Check sheet for the modelled part. Datum: model origin and axes. Units: mm. A direction names the side the tool comes from. Give positions to 0.01 mm unless a question says otherwise; leave off trailing zeros. Loops run counter-clockwise (first coordinate to the right, second up) from the corner with the lowest first, then second, coordinate; pieces in that order, holes last. Notation, with made-up numbers: (-8.75, 66) - (15.25, 66) arc R26 cw to (15.25, 101) - close; hole circle Ø1 at (27.25, 85.5). An arc over 180 degrees is marked (long way). Answer in a Markdown table with one row per item. Add a question column.
(1) Thickness scan on L1, parallel to Y at x = 0, z = -2.25; L2, parallel to Y at x = 0, z = 3.8; L3, parallel to Z at x = -14.75, y = 0. Record the ranges inside material, lowest first.
(2) Sectioned sample at C-C on z = 0.5. Enter the section's corners in (x, y), then the cut area to 3 significant figures.
(3) Set-up check for faces 1 (the face through (-2.39, -10.36, -4.93)), 2 (the face through (0.37, 7.34, 2.46)): record each of +Z, -Z, +X, -X, +Y, -Y from which the full face is reachable in a straight line by a thin tool's end or side.
(4) Go/stop test with flat-tipped pins: P1, Ø6, axis at x = -6, z = -4.5, coming from the -Y side; P2, Ø0.7, axis at x = -6, y = 1, coming from the -Z side; P3, Ø0.7, axis at x = -7, z = -5, coming from the -Y side. Record where each tip stops, or that it passes through.
(5) Draft check along Y on faces 3 (the face through (4, 0, -10)), 4 (the face through (2.39, 10.36, -4.93)). Enter one of: released by +Y, released by -Y, zero draft, split by the parting line, or undercut.
(6) Sectioned sample at A-A on y = 0. State how many separate pieces and enclosed holes the cut face has, then the cut area to 3 significant figures.
(7) Sectioned sample at B-B on x = 0. Enter the section's corners in (y, z), then the cut area to 3 significant figures.
from build123d import *

# Parameters (mm, degrees)
SKETCH1_R                           = 17.5
SKETCH1_R_2                         = 2.5
BOSS_EXTRUDE1_DEPTH                 = 10
BOSS_EXTRUDE2_START                 = 5
SKETCH1_3_R                         = 17.5
BOSS_EXTRUDE2_DEPTH                 = 5
M3_CLEARANCE_HOLE1_D                = 3.4
CUT_EXTRUDE1_REACH                  = 32.582
CUT_EXTRUDE1_END_RADIUS             = 17.5
SKETCH8_R                           = 1.5
CUT_EXTRUDE1_DIRECTION_2_REACH      = 32.582
CUT_EXTRUDE1_DIRECTION_2_END_RADIUS = 2.5
CUT_EXTRUDE2_DEPTH                  = 2.2


with BuildPart() as part:
    # Sketch1 → Boss-Extrude1 (new body)
    with BuildSketch(Plane.XY):
        Circle(SKETCH1_R)
        Circle(SKETCH1_R_2, mode=Mode.SUBTRACT)
        Polygon((1.58771324, 11.75), (-1.58771324, 11.75), (-3.175426481, 9), (-1.58771324, 6.25), (1.58771324, 6.25), (3.175426481, 9), align=None, mode=Mode.SUBTRACT)
        Polygon((1.58771324, -6.25), (-1.58771324, -6.25), (-3.175426481, -9), (-1.58771324, -11.75), (1.58771324, -11.75), (3.175426481, -9), align=None, mode=Mode.SUBTRACT)
    extrude(amount=-BOSS_EXTRUDE1_DEPTH)

    # Sketch1<3> → Boss-Extrude2 (add)
    with BuildSketch(Plane.XY.offset(BOSS_EXTRUDE2_START)):
        Circle(SKETCH1_3_R)
    extrude(amount=-BOSS_EXTRUDE2_DEPTH)

    # M3 Clearance Hole1 (through all)
    with Locations(Plane.XY.offset(5)):
        with Locations((0, 9), (0, -9)):
            Hole(M3_CLEARANCE_HOLE1_D / 2)

    # Cut-Extrude1: up to this cylinder (the profile starts inside it)
    cut_extrude1_end = Plane(origin=(0, 0, -5.7), z_dir=(0, 0, 1)) * Cylinder(CUT_EXTRUDE1_END_RADIUS, 101.164, mode=Mode.PRIVATE)
    # Sketch8 → Cut-Extrude1 (cut, up to the surface)
    with BuildSketch(Plane(origin=(5.5, 0, 0), x_dir=(0, 0, -1), z_dir=(1, 0, 0)), mode=Mode.PRIVATE) as cut_extrude1_sk1:
        with Locations((5.7, 0)):
            Circle(SKETCH8_R)
    cut_extrude1_tool1 = extrude(cut_extrude1_sk1.sketch, amount=CUT_EXTRUDE1_REACH, mode=Mode.PRIVATE) & cut_extrude1_end
    cut_extrude1 = cut_extrude1_tool1.solids().sort_by_distance((5.5, 0, -5.7))[0]
    add(cut_extrude1, mode=Mode.SUBTRACT)

    # Cut-Extrude1 direction 2: up to this cylinder (the profile starts outside it)
    cut_extrude1_direction_2_end = Plane(origin=(0, 0, -5.7), z_dir=(0, 0, 1)) * Cylinder(CUT_EXTRUDE1_DIRECTION_2_END_RADIUS, 71.164, mode=Mode.PRIVATE)
    # Sketch8 → Cut-Extrude1 direction 2 (cut, up to the surface)
    with BuildSketch(Plane(origin=(5.5, 0, 0), x_dir=(0, 0, -1), z_dir=(1, 0, 0)), mode=Mode.PRIVATE) as cut_extrude1_direction_2_sk1:
        with Locations((5.7, 0)):
            Circle(SKETCH8_R)
    cut_extrude1_direction_2_tool1 = extrude(cut_extrude1_direction_2_sk1.sketch, amount=-CUT_EXTRUDE1_DIRECTION_2_REACH, mode=Mode.PRIVATE) - cut_extrude1_direction_2_end
    cut_extrude1_direction_2 = cut_extrude1_direction_2_tool1.solids().sort_by_distance((5.5, 0, -5.7))[0]
    add(cut_extrude1_direction_2, mode=Mode.SUBTRACT)
    cut_extrude1 = cut_extrude1 + cut_extrude1_direction_2  # both directions under the feature's name, for the pattern or mirror that repeats it

    # Sketch8<4> → Cut-Extrude2 (cut)
    with BuildSketch(Plane(origin=(5.5, 0, 0), x_dir=(0, 0, -1), z_dir=(1, 0, 0))):
        Polygon((8.5, 2.8), (2.9, 2.8), (2.9, -2.8), (8.5, -2.8), (10, -2.8), (10, 2.8), align=None)
    cut_extrude2 = extrude(amount=CUT_EXTRUDE2_DEPTH, mode=Mode.SUBTRACT)

    # Mirror1: Cut-Extrude1, Cut-Extrude2 across plane
    add(cut_extrude1.mirror(Plane(origin=(0, 0, 0), x_dir=(0, 0, 1), z_dir=(1, 0, 0))), mode=Mode.SUBTRACT)
    add(cut_extrude2.mirror(Plane(origin=(0, 0, 0), x_dir=(0, 0, 1), z_dir=(1, 0, 0))), mode=Mode.SUBTRACT)


solid = part.part
Reply:
| question | item | result |
|---|---|---|
| 1 | L1 | -17.5 to -11.75, -6.25 to -2.5, 2.5 to 6.25, 11.75 to 17.5 |
| 1 | L2 | -17.5 to -10.7, -7.3 to 7.3, 10.7 to 17.5 |
| 1 | L3 | -10 to -7.2, -4.2 to 5 |
| 2 | outline | circle Ø35 at (0, 0); hole circle Ø3.4 at (0, -9); hole circle Ø3.4 at (0, 9) |
| 2 | area | 944 mm^2 |
| 3 | face 1 | -Z |
| 3 | face 2 | +Z, -Z |
| 4 | P1 | y = -17.24 |
| 4 | P2 | z = -2.9 |
| 4 | P3 | y = -16.19 |
| 5 | face 3 | zero draft |
| 5 | face 4 | undercut |
| 6 | separate pieces | 5 |
| 6 | enclosed holes | 0 |
| 6 | area | 367 mm^2 |
| 7 | outline | (-17.5, -10) - (-11.75, -10) - (-11.75, 0) - (-10.7, 0) - (-10.7, 5) - (-17.5, 5) - close; (-7.3, 0) - (-6.25, 0) - (-6.25, -10) - (-2.5, -10) - (-2.5, 0) - (2.5, 0) - (2.5, -10) - (6.25, -10) - (6.25, 0) - (7.3, 0) - (7.3, 5) - (-7.3, 5) - close; (10.7, 0) - (11.75, 0) - (11.75, -10) - (17.5, -10) - (17.5, 5) - (10.7, 5) - close |
| 7 | area | 331 mm^2 |
